from build123d import *

# Parameters (mm, degrees)
SKETCH1_R               = 6.35
BOSS_EXTRUDE1_DEPTH     = 8.382
SKETCH6_W               = 8.382
SKETCH6_H               = 10.16
BOSS_EXTRUDE2_DEPTH     = 31.75
CUT_EXTRUDE4_DEPTH      = 37.592
BOSS_EXTRUDE3_START     = -8.382
BOSS_EXTRUDE3_DEPTH     = 8.382
BOSS_EXTRUDE4_START     = -8.382
SKETCH11_R              = 6.35
BOSS_EXTRUDE4_DEPTH     = 8.382
FILLET1_R               = 2.54
CUT_EXTRUDE5_DEPTH      = 12.192
CUT_EXTRUDE6_DEPTH      = 2.54
CUT_EXTRUDE6_DEPTH_BACK = 45.396714307
SKETCH13_W              = 3.302
SKETCH13_H              = 3.81
CUT_EXTRUDE7_DEPTH      = 5.842
CUT_EXTRUDE7_DEPTH_BACK = 2.032
SKETCH14_W              = 2.286
SKETCH14_H              = 39.733795437
BOSS_EXTRUDE5_DEPTH     = 2.286
SKETCH19_R              = 4.572
CUT_EXTRUDE8_DEPTH      = 20.32
CHAMFER1_SIZE           = 2.54
CHAMFER1_SIZE_2         = 1.929900828


with BuildPart() as part:
    # Sketch1 → Boss-Extrude1 (new body)
    with BuildSketch(Plane(origin=(0, 0, 0), x_dir=(0, 0, -1), z_dir=(1, 0, 0))):
        Circle(SKETCH1_R)
    extrude(amount=BOSS_EXTRUDE1_DEPTH)

    # Sketch6 → Boss-Extrude2 (add)
    with BuildSketch(Plane.XY):
        with Locations((4.191, 0)):
            Rectangle(SKETCH6_W, SKETCH6_H)
    extrude(amount=BOSS_EXTRUDE2_DEPTH)

    # Sketch9 → Cut-Extrude4 (cut)
    with BuildSketch(Plane.ZY):
        with BuildLine():
            Line((31.75, 5.08), (11.408365483, 5.08))
            Line((11.408365483, 5.08), (3.81, 5.08))
            ThreePointArc((3.81, 5.08), (5.339430543, 3.232524289), (6.092803339, 0.955518862))
            Line((6.092803339, 0.955518862), (11.408365483, 0.955518862))
            Line((11.408365483, 0.955518862), (11.408365483, -5.08))
            Line((11.408365483, -5.08), (31.75, -5.08))
            Line((31.75, -5.08), (31.75, 5.08))
        make_face()
    extrude(amount=-CUT_EXTRUDE4_DEPTH, mode=Mode.SUBTRACT)

    # Sketch8 → Boss-Extrude3 (add)
    with BuildSketch(Plane(origin=(8.382, 0, 0), x_dir=(0, 0, -1), z_dir=(1, 0, 0)).offset(BOSS_EXTRUDE3_START)):
        with BuildLine():
            ThreePointArc((-4.292149369, 4.679738646), (-6.310240248, 0.709484333), (-5.22417178, -3.609782433))
            ThreePointArc((-5.22417178, -3.609782433), (-6.393298566, -4.253843839), (-7.59869899, -4.827152092))
            ThreePointArc((-7.59869899, -4.827152092), (-24.920173533, -6.389046133), (-41.525963587, -1.219836328))
            ThreePointArc((-41.525963587, -1.219836328), (-41.809620195, 1.017710808), (-40.915378479, 3.088317002))
            ThreePointArc((-40.915378479, 3.088317002), (-22.743048705, 7.089374731), (-4.292149369, 4.679738646))
        make_face()
    extrude(amount=BOSS_EXTRUDE3_DEPTH)

    # Sketch11 → Boss-Extrude4 (add)
    with BuildSketch(Plane(origin=(8.382, 0, 0), x_dir=(0, 0, -1), z_dir=(1, 0, 0)).offset(BOSS_EXTRUDE4_START)):
        Circle(SKETCH11_R)
    extrude(amount=BOSS_EXTRUDE4_DEPTH)

    # Fillet1
    fillet1_edges = [part.edges().sort_by_distance(p)[0] for p in [
        (4.191, -1.219836328, 41.525963587),
        (4.191, 3.088317002, 40.915378479),
    ]]
    fillet(fillet1_edges, radius=FILLET1_R)

    # Sketch12 → Cut-Extrude5 (cut)
    with BuildSketch(Plane.ZY):
        with BuildLine():
            Line((5.311349681, -3.480239153), (6.475883823, -5.08))
            Line((6.475883823, -5.08), (3.81, -5.08))
            ThreePointArc((3.81, -5.08), (4.630287647, -4.345450069), (5.311349681, -3.480239153))
        make_face()
    extrude(amount=-CUT_EXTRUDE5_DEPTH, mode=Mode.SUBTRACT)

    # Sketch13 → Cut-Extrude6 (cut, two sides: drawn at the far end of the back side and taken through both)
    with BuildSketch(Plane.XZ.offset(5.08).offset(-CUT_EXTRUDE6_DEPTH_BACK)):
        with Locations((4.191, 30.937666225)):
            Rectangle(SKETCH13_W, SKETCH13_H)
        with Locations((4.191, 22.047666225)):
            Rectangle(SKETCH13_W, SKETCH13_H)
    extrude(amount=CUT_EXTRUDE6_DEPTH + CUT_EXTRUDE6_DEPTH_BACK, mode=Mode.SUBTRACT)

    # Sketch14 → Cut-Extrude7 (cut, two sides: drawn at the far end of the back side and taken through both)
    with BuildSketch(Plane.XZ.offset(5.08).offset(-CUT_EXTRUDE7_DEPTH_BACK)):
        with Locations((4.191, 9.165768507)):
            Rectangle(SKETCH14_W, SKETCH14_H)
    extrude(amount=CUT_EXTRUDE7_DEPTH + CUT_EXTRUDE7_DEPTH_BACK, mode=Mode.SUBTRACT)

    # Sketch15 → Boss-Extrude5 (add)
    with BuildSketch(Plane.ZY.offset(-5.334)):
        with BuildLine():
            Line((20.142666225, -3.048), (5.311349681, -4.064))
            ThreePointArc((5.311349681, -4.064), (0.047585795, -5.585594771), (-4.808654899, -3.048))
            Line((-4.808654899, -3.048), (20.142666225, -3.048))
        make_face()
    extrude(amount=BOSS_EXTRUDE5_DEPTH)

    # Sketch19 → Cut-Extrude8 (cut)
    with BuildSketch(Plane(origin=(8.382, 0, 0), x_dir=(0, 0, -1), z_dir=(1, 0, 0))):
        Circle(SKETCH19_R)
    extrude(amount=-CUT_EXTRUDE8_DEPTH, mode=Mode.SUBTRACT)

    # Chamfer1
    # the kernel refuses this chamfer: 2.54, 1.929900828 mm, written as the material it takes off along each edge
    with BuildSketch(Plane(origin=(-6.584556216, -5.08, 6.475883823), x_dir=(0, 0.7995159790431987, -0.6006448195519506), z_dir=(1, 0, 0))) as chamfer1_piece_1_section:
        Polygon((CHAMFER1_SIZE * 0.999886403459, CHAMFER1_SIZE * 0.0150724974299), (-CHAMFER1_SIZE_2 * 0.600644819472, CHAMFER1_SIZE_2 * 0.799515978937), (0, 0), align=None)
    chamfer1_piece_1 = extrude(amount=9.632556216, mode=Mode.PRIVATE)
    chamfer1_piece_1 = chamfer1_piece_1 - Plane(origin=(1.524, 0, 0), x_dir=(0, -0.800000000000003, 0.5999999999999959), z_dir=(-1, 0, 0)) * Cylinder(6.35, 30, mode=Mode.PRIVATE)
    add(chamfer1_piece_1, mode=Mode.SUBTRACT)
    with BuildSketch(Plane(origin=(-6.584556216, -5.08, 6.475883823), x_dir=(0, 0.7995159790431987, -0.6006448195519506), z_dir=(1, 0, 0))) as chamfer1_piece_2_section:
        Polygon((CHAMFER1_SIZE * 0.999886403459, CHAMFER1_SIZE * 0.0150724974299), (-CHAMFER1_SIZE_2 * 0.600644819472, CHAMFER1_SIZE_2 * 0.799515978937), (0, 0), align=None)
    chamfer1_piece_2 = extrude(amount=16.217112431, mode=Mode.PRIVATE)
    chamfer1_piece_2 = chamfer1_piece_2 - Plane(origin=(6.858, 0, 0), x_dir=(0, -0.800000000000003, 0.5999999999999959), z_dir=(-1, 0, 0)) * Cylinder(6.35, 43, mode=Mode.PRIVATE)
    chamfer1_piece_2 = split(chamfer1_piece_2, bisect_by=Plane(origin=(5.334, -3.740270515, 5.829817166), z_dir=(1, 0, 0)), keep=Keep.TOP, mode=Mode.PRIVATE)
    add(chamfer1_piece_2, mode=Mode.SUBTRACT)
    with BuildSketch(Plane(origin=(-1.250556216, -5.08, 6.475883823), x_dir=(0, 0.7995159790431987, -0.6006448195519506), z_dir=(1, 0, 0))) as chamfer1_piece_3_section:
        Polygon((CHAMFER1_SIZE * 0.999886403459, CHAMFER1_SIZE * 0.0150724974299), (-CHAMFER1_SIZE_2 * 0.600644819472, CHAMFER1_SIZE_2 * 0.799515978937), (0, 0), align=None)
    chamfer1_piece_3 = extrude(amount=16.217112431, mode=Mode.PRIVATE)
    chamfer1_piece_3 = chamfer1_piece_3 - Plane(origin=(1.524, 0, 0), x_dir=(0, -0.800000000000003, 0.5999999999999959), z_dir=(-1, 0, 0)) * Cylinder(6.35, 43, mode=Mode.PRIVATE)
    chamfer1_piece_3 = split(chamfer1_piece_3, bisect_by=Plane(origin=(3.048, -3.740270515, 5.829817166), z_dir=(-1, 0, 0)), keep=Keep.TOP, mode=Mode.PRIVATE)
    add(chamfer1_piece_3, mode=Mode.SUBTRACT)
    with BuildSketch(Plane(origin=(5.334, -5.08, 6.475883823), x_dir=(0, 0.7995159790431987, -0.6006448195519506), z_dir=(1, 0, 0))) as chamfer1_piece_4_section:
        Polygon((CHAMFER1_SIZE * 0.999886403459, CHAMFER1_SIZE * 0.0150724974299), (-CHAMFER1_SIZE_2 * 0.600644819472, CHAMFER1_SIZE_2 * 0.799515978937), (0, 0), align=None)
    chamfer1_piece_4 = extrude(amount=9.632556216, mode=Mode.PRIVATE)
    chamfer1_piece_4 = chamfer1_piece_4 - Plane(origin=(6.858, 0, 0), x_dir=(0, -0.800000000000003, 0.5999999999999959), z_dir=(-1, 0, 0)) * Cylinder(6.35, 30, mode=Mode.PRIVATE)
    add(chamfer1_piece_4, mode=Mode.SUBTRACT)


solid = part.part
For this review, take the finished solid that the model builds, in its own axes (mm). A direction names the side the tool comes from. Round coordinates to 2 decimals unless told otherwise and drop trailing zeros. Loops run counter-clockwise (first coordinate to the right, second up) from the corner with the lowest first, then second, coordinate; pieces in that order, holes last. Notation, with made-up numbers: (28.5, 31) - (66.5, 31) arc R23 cw to (66.5, 39) - close; hole circle Ø7 at (-7.75, 14). An arc over 180 degrees is marked (long way). One line per item, written item: value. Start each with the question number.
Item 1: The part is to be moulded in two halves that separate along Z. For faces 5 (the cylindrical face through (4.132, 1.271, 41.766)), 6 (the flat face through (5.334, -5, 26)), 7 (the flat face through (3.048, -5.5, -1.8)), say which applies: +Z half, -Z half, draft (parallel to the pull), parting line (faces both ways), or undercut.
Item 2: Take a section at D-D (z = 38). Give the boundary of the cut face in (x, y), plus the area to 3 significant figures.
Item 3: Clearance check with flat-ended pins moving along their axes: pin 1 Ø1 at (x, z) = (5.5, 25) entering from -Y; pin 2 Ø0.8 at (x, z) = (4, -5.5) entering from -Y; pin 3 Ø3.5 at (x, y) = (3.5, 2) entering from -Z. State where each tip first meets the part, or that it passes through.
Item 4: For L1, parallel to Y at x = 6.5, z = 0; L2, parallel to Z at x = 4.5, y = 2.25; L3, parallel to X at y = 1, z = 32, list the stretches that pass through material, from the lowest coordinate up.
Item 5: For faces 1 (the flat face through (6.837, -4.175, 6.896)), 2 (the flat face through (4, 2, 20.143)), 3 (the flat face through (4, -3.048, 27)), 4 (the flat face through (1.503, -4.175, 6.896)), list the 3-axis set-ups (+Z, -Z, +X, -X, +Y, -Y) from which the entire face can be reached by the end or side of a thin tool; tool diameter is ignored.
Item 6: Take a section at B-B (y = 5.25). Give the boundary of the cut face in (x, z).
Item 7: Take a section at C-C (z = 25.5). Give the boundary of the cut face in (x, y).
Item 8: Take a section at A-A (z = 0). Give the boundary of the cut face in (x, y).
Answer below:
1. face 5: +Z half
1. face 6: undercut
1. face 7: draft
2. outline: (0, -2.94) - (8.38, -2.94) - (8.38, 4.19) - (0, 4.19) - close
2. area: 59.8 mm2
3. pin 1: stops at y = -6.43
3. pin 2: stops at y = -3.05
3. pin 3: stops at z = -6.35
4. L1: y = -6.35 to -4.57, 4.57 to 6.35
4. L2: z = -5.94 to -3.98, 3.98 to 20.14, 23.95 to 29.03, 32.84 to 41.43
4. L3: x = 0 to 2.54, 5.84 to 8.38
5. face 1: +X, -Y
5. face 2: +Y, -Y
5. face 3: -Y
5. face 4: -X, -Y
6. outline: (0, -3.57) - (8.38, -3.57) - (8.38, 3.57) - (0, 3.57) - close; (0, 6.24) - (8.38, 6.24) - (8.38, 34.56) - (0, 34.56) - close; hole (2.54, 20.14) - (5.84, 20.14) - (5.84, 23.95) - (2.54, 23.95) - close; hole (2.54, 29.03) - (5.84, 29.03) - (5.84, 32.84) - (2.54, 32.84) - close
7. outline: (0, -6.32) - (3.05, -6.32) - (3.05, -3.05) - (5.33, -3.05) - (5.33, -6.32) - (8.38, -6.32) - (8.38, 6.9) - (0, 6.9) - close
8. outline: (0, -6.35) - (3.05, -6.35) - (3.05, -5.58) - (5.33, -5.58) - (5.33, -6.35) - (8.38, -6.35) - (8.38, -4.57) - (0, -4.57) - close; (0, 4.57) - (8.38, 4.57) - (8.38, 6.35) - (0, 6.35) - close
